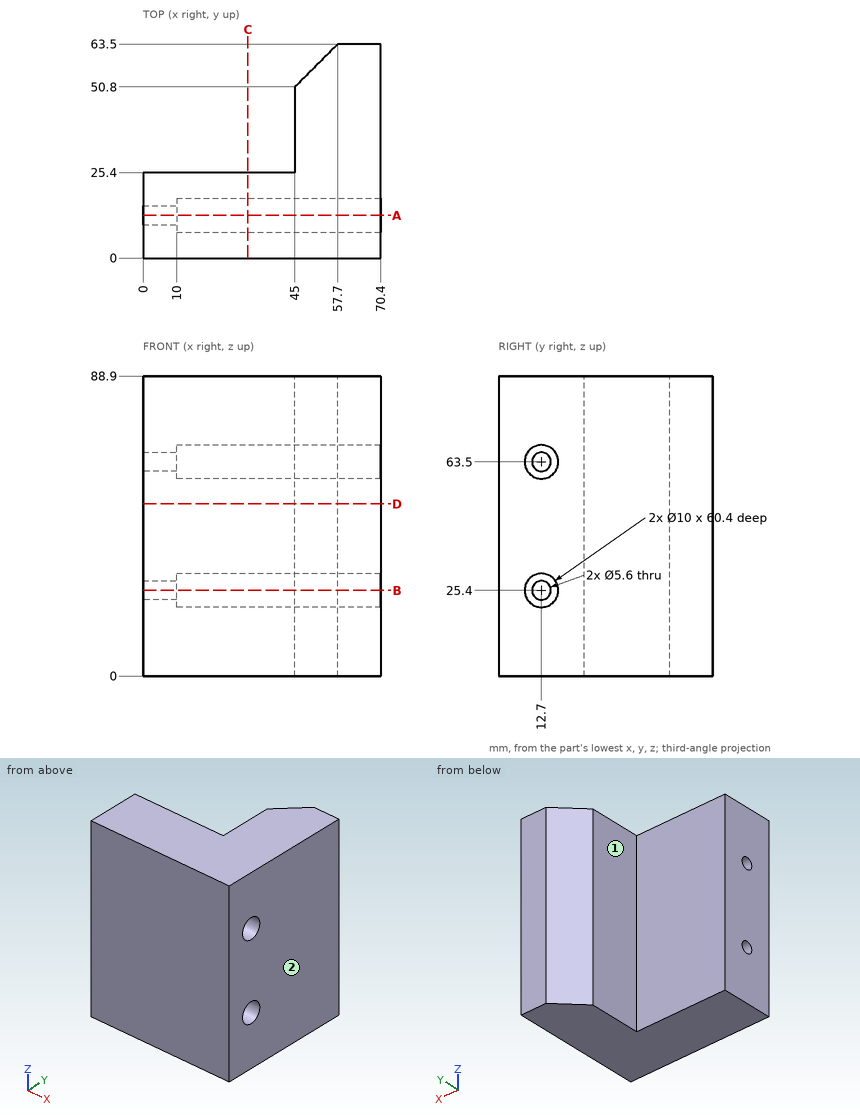
Input: dimensioned drawing with shaded views. Units: mm. Origin: part minimum x, y, z. A direction names the side the tool comes from. Round coordinates to 2 decimals unless told otherwise and drop trailing zeros. Order: outer loops, then holes, each group sorted by start corner. A loop starts at its lowest first (then second) coordinate and runs counter-clockwise, first axis right, second up.
1. Pin query (flat end, axial travel): P1, Ø7.5, axis at y = 12.7, z = 25.4, coming from the +X side; P2, Ø1.5, axis at y = 42, z = 78, coming from the -X side. Return the tip coordinate at first contact, or that it passes through.
The answers:
P1: stops at x = 10
P2: stops at x = 45
2. Cut plane D-D, the plane z = 51. Output: boundary loops of the cut face in (x, y).
The answers:
outline: (0, 0) - (70.4, 0) - (70.4, 63.5) - (57.7, 63.5) - (45, 50.8) - (45, 25.4) - (0, 25.4) - close
3. Cut plane B-B, the plane z = 25.4. Output: boundary loops of the cut face in (x, y).
The answers:
outline: (0, 0) - (70.4, 0) - (70.4, 7.7) - (10, 7.7) - (10, 9.9) - (0, 9.9) - close; (0, 15.5) - (10, 15.5) - (10, 17.7) - (70.4, 17.7) - (70.4, 63.5) - (57.7, 63.5) - (45, 50.8) - (45, 25.4) - (0, 25.4) - close
4. Material intervals for line 1 (Y direction, x = 8, z = 25.4); line 2 (Z direction, x = 61, y = 16); line 3 (Y direction, x = 40, z = 40.5), sorted ascending.
The answers:
line 1: y = 0 to 9.9, 15.5 to 25.4
line 2: z = 0 to 21.64, 29.16 to 59.74, 67.26 to 88.9
line 3: y = 0 to 25.4
5. Set-up query: the marked faces 1 and 2. Return all of +Z, -Z, +X, -X, +Y, -Y with unobstructed straight access to the full face (end or side cutting, diameter ignored); none if empty.
The answers:
face 1: +Z, -Z, -X, +Y
face 2: +Z, -Z, +X, +Y, -Y
6. Cut plane A-A, the plane y = 12.7. Output: boundary loops of the cut face in (x, z), then the cut area to 3 significant figures.
The answers:
outline: (0, 0) - (70.4, 0) - (70.4, 20.4) - (10, 20.4) - (10, 22.6) - (0, 22.6) - close; (0, 28.2) - (10, 28.2) - (10, 30.4) - (70.4, 30.4) - (70.4, 58.5) - (10, 58.5) - (10, 60.7) - (0, 60.7) - close; (0, 66.3) - (10, 66.3) - (10, 68.5) - (70.4, 68.5) - (70.4, 88.9) - (0, 88.9) - close
area: 4,940 mm2
7. Cut plane C-C, the plane x = 31. Output: boundary loops of the cut face in (y, z).
The answers:
outline: (0, 0) - (25.4, 0) - (25.4, 88.9) - (0, 88.9) - close; hole circle Ø10 at (12.7, 25.4); hole circle Ø10 at (12.7, 63.5)
